```python
from build123d import *

# Parameters (mm, degrees)
SKETCH_1_R          = 1.5
SKETCH_1_W          = 7
SKETCH_1_H          = 7
EXTRUDE_1_DEPTH     = 4
CUT_EXTRUDE_1_DEPTH = 5
FILLET_1_R          = 10
CHAMFER_1_SIZE      = 1.5


with BuildPart() as part:
    # Эскиз1 → Бобышка-Вытянуть1 (new body)
    with BuildSketch(Plane.XY):
        with BuildLine():
            Line((7.5, -9.463206067), (-7.5, -9.463206067))
            Line((-7.5, -9.463206067), (-7.5, 3.572357891))
            ThreePointArc((-7.5, 3.572357891), (-14.05213631, 6.841981187), (-7.21473133, 9.463206067))
            Line((-7.21473133, 9.463206067), (7.5, 9.463206067))
            Line((7.5, 9.463206067), (7.5, -0.443591232))
            ThreePointArc((7.5, -0.443591232), (11.733092656, -4.436793933), (7.5, -8.429996634))
            Line((7.5, -8.429996634), (7.5, -9.463206067))
        make_face()
        with Locations((7.733092656, -4.436793933)):
            Circle(SKETCH_1_R, mode=Mode.SUBTRACT)
        with Locations((-10.056818182, 6.648504959)):
            Circle(SKETCH_1_R, mode=Mode.SUBTRACT)
        with Locations((-1.5, 0.563206067)):
            Rectangle(SKETCH_1_W, SKETCH_1_H, mode=Mode.SUBTRACT)
    extrude(amount=EXTRUDE_1_DEPTH)

    # Эскиз2 → Вырез-Вытянуть1 (cut, through all)
    with BuildSketch(Plane(origin=(0, 0, 0), x_dir=(-1, 0, 0), z_dir=(0, 0, -1))):
        with BuildLine():
            Line((7.5, -9.463206067), (-7.5, -9.463206067))
            Line((-7.5, -9.463206067), (-7.5, -8.429996634))
            ThreePointArc((-7.5, -8.429996634), (-6.727483224, -8.308324595), (-5.993405004, -8.038666623))
            ThreePointArc((-5.993405004, -8.038666623), (-5.272781318, -8.335553846), (-4.5, -8.436793933))
            Line((-4.5, -8.436793933), (7.5, -8.436793933))
            Line((7.5, -8.436793933), (7.5, -9.463206067))
        make_face()
    extrude(amount=-CUT_EXTRUDE_1_DEPTH, mode=Mode.SUBTRACT)

    # Скругление1
    fillet_1_edges = [part.edges().sort_by_distance(p)[0] for p in [
        (-7.5, 3.572357891, 2),
    ]]
    fillet(fillet_1_edges, radius=FILLET_1_R)

    # Фаска1
    chamfer_1_edges = [part.edges().sort_by_distance(p)[0] for p in [
        (6.233092656, -4.436793933, 0),
        (-11.556818182, 6.648504959, 0),
    ]]
    chamfer(chamfer_1_edges, length=CHAMFER_1_SIZE)


solid = part.part
```
Here's how the part is built. I have some questions about the finished solid (model axes, mm). A direction names the side the tool comes from. Coordinates: 2 decimals unless noted, no trailing zeros. Loops run counter-clockwise (first coordinate to the right, second up) from the corner with the lowest first, then second, coordinate; pieces in that order, holes last. Notation, with made-up numbers: (0.25, -9) - (25.25, -9) arc R13 ccw to (25.25, 3) - close; hole circle Ø7 at (20.25, 62.5). An arc over 180 degrees is marked (long way). Return JSON: item names as keys, results as strings. Group by question number.
Item 1: On a 3-axis mill with a long thin cutter (end or side, diameter ignored), from which of +Z, -Z, +X, -X, +Y, -Y can I reach the whole of each face in a straight line? I mean faces 1 (the face through (-2, -2.937, 2)), 2 (the face through (7.5, 5, 2)), 3 (the face through (5.283, -8.333, 1.972)), 4 (the face through (-7.5, -7, 2)). Say none if no direction works.
Item 2: Will these pins go through, and if not, where does the flat tip stop? P1, Ø1.2, axis at x = -0.5, z = 1, coming from the +Y side; P2, Ø1.2, axis at y = 6.5, z = 2, coming from the +X side; P3, Ø5, axis at x = -10.06, y = 6.65, coming from the -Z side.
Item 3: If we section it at C-C on z = 3.3: Write out the boundary of the cut face in (x, y).
Item 4: If we section it at A-A on x = 1.25: Write out the boundary of the cut face in (y, z), and give its area (3 significant figures).
Item 5: I need wall thicknesses on line 1 (X direction, y = 6.75, z = 1.9); line 2 (Y direction, x = -1, z = 0.8); line 3 (X direction, y = -4, z = 1.65). Which ranges of each line are inside material? Lowest first, please. Write a range as from..to.
Item 6: If we section it at B-B on y = 0: Write out the boundary of the cut face in (x, z), and give its area (3 significant figures).
Item 7: We'd pull the mould along X, two halves only. Please class faces 5 (the face through (6.63, -3.42, 2.73)), 6 (the face through (-8.78, -0.31, 2.03)), 7 (the face through (-13.24, 9.07, 1.97)): +X half, -X half, draft (parallel to the pull), parting line (faces both ways), or undercut.
Calculated:
{
 "1": {"face 1": "+Z, -Z", "face 2": "+Z, -Z, +X, +Y", "face 3": "+Z, -Z, -Y", "face 4": "+Z, -Z, -X, -Y"},
 "2": {"P1": "stops at y = 9.46", "P2": "stops at x = 7.5", "P3": "stops at z = 0.5"},
 "3": {"outline": "(-12.18, 3.26) arc R10 cw to (-7.5, -5.21) - (-7.5, -8.44) - (4.5, -8.44) arc R3 ccw to (5.99, -8.04) arc R4 ccw (long way) to (7.5, -0.44) - (7.5, 9.46) - (-7.21, 9.46) arc R4 ccw (long way) to start; hole circle Ø3 at (-10.06, 6.65); hole (-5, -2.94) - (2, -2.94) - (2, 4.06) - (-5, 4.06) - close; hole circle Ø3 at (7.73, -4.44)"},
 "4": {"outline": "(-8.44, 0) - (-2.94, 0) - (-2.94, 4) - (-8.44, 4) - close; (4.06, 0) - (9.46, 0) - (9.46, 4) - (4.06, 4) - close", "area": "43.6 mm^2"},
 "5": {"line 1": "x = -14.06..-11.55, -8.56..7.5", "line 2": "y = -8.44..-2.94, 4.06..9.46", "line 3": "x = -7.57..6.3, 9.17..11.71"},
 "6": {"outline": "(-8.96, 0) - (-5, 0) - (-5, 4) - (-8.96, 4) - close; (2, 0) - (7.5, 0) - (7.5, 4) - (2, 4) - close", "area": "37.9 mm^2"},
 "7": {"face 5": "undercut", "face 6": "-X half", "face 7": "parting line"}
}
